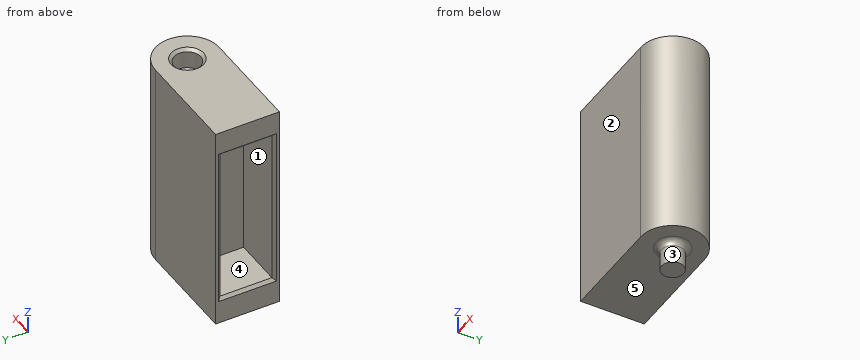
from build123d import *

# Parameters (mm, degrees)
BOSS_EXTRU_1_DEPTH      = 36
ESQUISSE2_W             = 27
ESQUISSE2_H             = 9
ENL_V_MAT_EXTRU_1_DEPTH = 9
ESQUISSE3_R             = 2.3
ENL_V_MAT_EXTRU_2_DEPTH = 3.5
ESQUISSE4_R             = 1.9
BOSS_EXTRU_2_DEPTH      = 4.1
CONG_1_R                = 1
CHANFREIN1_SIZE         = 0.5
CHANFREIN2_SIZE         = 0.5


with BuildPart() as part:
    # Esquisse1 → Boss.-Extru.1 (new body)
    with BuildSketch(Plane.XY):
        with BuildLine():
            Line((0, 5.5), (-18, 5.5))
            Line((-18, 5.5), (-18, -5.5))
            Line((-18, -5.5), (0, -5.5))
            ThreePointArc((0, -5.5), (5.5, 0), (0, 5.5))
        make_face()
    extrude(amount=BOSS_EXTRU_1_DEPTH)

    # Esquisse2 → Enlèv. mat.-Extru.1 (cut)
    with BuildSketch(Plane.ZY.offset(18)):
        with Locations((18.047533914, 0)):
            Rectangle(ESQUISSE2_W, ESQUISSE2_H)
    extrude(amount=-ENL_V_MAT_EXTRU_1_DEPTH, mode=Mode.SUBTRACT)

    # Esquisse3 → Enlèv. mat.-Extru.2 (cut)
    with BuildSketch(Plane.XY.offset(36)):
        Circle(ESQUISSE3_R)
    extrude(amount=-ENL_V_MAT_EXTRU_2_DEPTH, mode=Mode.SUBTRACT)

    # Esquisse4 → Boss.-Extru.2 (add)
    with BuildSketch(Plane(origin=(0, 0, 0), x_dir=(-1, 0, 0), z_dir=(0, 0, -1))):
        with Locations(Location((0, 0, 0), (0, 0, 180))):
            Circle(ESQUISSE4_R)
    extrude(amount=BOSS_EXTRU_2_DEPTH)

    # Congé1
    cong_1_edges = [part.edges().sort_by_distance(p)[0] for p in [
        (-1.9, 0, 0),
    ]]
    fillet(cong_1_edges, radius=CONG_1_R)

    # Chanfrein1
    chanfrein1_edges = [part.edges().sort_by_distance(p)[0] for p in [
        (-2.3, 0, 36),
    ]]
    chamfer(chanfrein1_edges, length=CHANFREIN1_SIZE)

    # Chanfrein2
    chanfrein2_edges = [part.edges().sort_by_distance(p)[0] for p in [
        (-18, 0, 4.547533914),
        (-18, -4.5, 18.047533914),
        (-18, 0, 31.547533914),
        (-18, 4.5, 18.047533914),
    ]]
    chamfer(chanfrein2_edges, length=CHANFREIN2_SIZE)


solid = part.part
The model under review builds one solid part; all positions refer to its coordinate system, in mm. Face numbers are marked on the shaded views. A direction names the side the tool comes from. Round coordinates to 2 decimals unless told otherwise and drop trailing zeros. Loops run counter-clockwise (first coordinate to the right, second up) from the corner with the lowest first, then second, coordinate; pieces in that order, holes last. Notation, with made-up numbers: (22, 28) -> (50, 28) arc R20 cw to (50, 48) -> close; hole circle Ø10 at (-7, -15.5). An arc over 180 degrees is marked (long way). Write item = value, one per line. Start each with the question number.
Item 1: For the marked faces 1 and 2, list the 3-axis set-ups (+Z, -Z, +X, -X, +Y, -Y) from which the entire face can be reached by the end or side of a thin tool; tool diameter is ignored.
Item 2: To check wall thickness, follow L1, parallel to Y at x = 0, z = 34.2; L2, parallel to Y at x = -12.75, z = 16.5; L3, parallel to Z at x = -16, y = 3.5. State the ranges of each line that lie inside material, in increasing order.
Item 3: Take a section at D-D on x = -3.75. Give the boundary of the cut face in (y, z), plus the area to 3 significant figures.
Item 4: Take a section at B-B on y = 0. Give the boundary of the cut face in (x, z).
Item 5: Take a section at C-C on z = 11.5. Give the boundary of the cut face in (x, y).
Item 6: Mouldability with a two-part tool opening along Z and no side actions: class the marked faces 3, 4 and 5 as released by +Z, released by -Z, zero draft, split by the parting line, or undercut.
Item 7: Take a section at A-A on x = -14.5. Give the boundary of the cut face in (y, z), plus the area to 3 significant figures.
Item 8: Insertion check: pin 1 (5 mm diameter, centred on y = 3, z = 16.5, fed in from +X); pin 2 (4.5 mm diameter, centred on y = 1, z = 12.5, fed in from -X); pin 3 (6 mm diameter, centred on y = 3, z = 5, fed in from -X); pin 4 (2.5 mm diameter, centred on x = 1, y = 1, fed in from +Z). Each pin has a flat end and moves straight along its axis. Give the tip position at first contact, or say it passes through.
Result:
q1.face_1 = -X
q1.face_2 = +Z, -Z, +X, -X, -Y
q2.L1 = -5.5 to -2.3, 2.3 to 5.5
q2.L2 = -5.5 to -4.5, 4.5 to 5.5
q2.L3 = 0 to 4.55, 31.55 to 36
q3.outline = (-5.5, 0) -> (5.5, 0) -> (5.5, 36) -> (-5.5, 36) -> close
q3.area = 396 mm²
q4.outline = (-18, 0) -> (-2.9, 0) arc R1 cw to (-1.9, -1) -> (-1.9, -4.1) -> (1.9, -4.1) -> (1.9, -1) arc R1 cw to (2.9, 0) -> (5.5, 0) -> (5.5, 36) -> (2.8, 36) -> (2.3, 35.5) -> (2.3, 32.5) -> (-2.3, 32.5) -> (-2.3, 35.5) -> (-2.8, 36) -> (-18, 36) -> (-18, 32.05) -> (-17.5, 31.55) -> (-9, 31.55) -> (-9, 4.55) -> (-17.5, 4.55) -> (-18, 4.05) -> close
q5.outline = (-18, -5.5) -> (0, -5.5) arc R5.5 ccw to (0, 5.5) -> (-18, 5.5) -> (-18, 5) -> (-17.5, 4.5) -> (-9, 4.5) -> (-9, -4.5) -> (-17.5, -4.5) -> (-18, -5) -> close
q6.face_3 = zero draft
q6.face_4 = undercut
q6.face_5 = released by -Z
q7.outline = (-5.5, 0) -> (5.5, 0) -> (5.5, 36) -> (-5.5, 36) -> close; hole (-4.5, 4.55) -> (4.5, 4.55) -> (4.5, 31.55) -> (-4.5, 31.55) -> close
q7.area = 153 mm²
q8.pin_1 = 5.48
q8.pin_2 = -9
q8.pin_3 = -18
q8.pin_4 = 35.86
